Source: three-view drawing plus pictorial views. Frame: mm from the lowest corner of the part. A direction names the side the tool comes from. Give positions to 0.01 mm unless a question says otherwise; leave off trailing zeros. Loops run counter-clockwise (first coordinate to the right, second up) from the corner with the lowest first, then second, coordinate; pieces in that order, holes last. Notation, with made-up numbers: (-25.75, 75) - (-19.75, 75) arc R18 cw to (-19.75, 107) - close; hole circle Ø5 at (19, -17). An arc over 180 degrees is marked (long way). One line per item, written item: value.
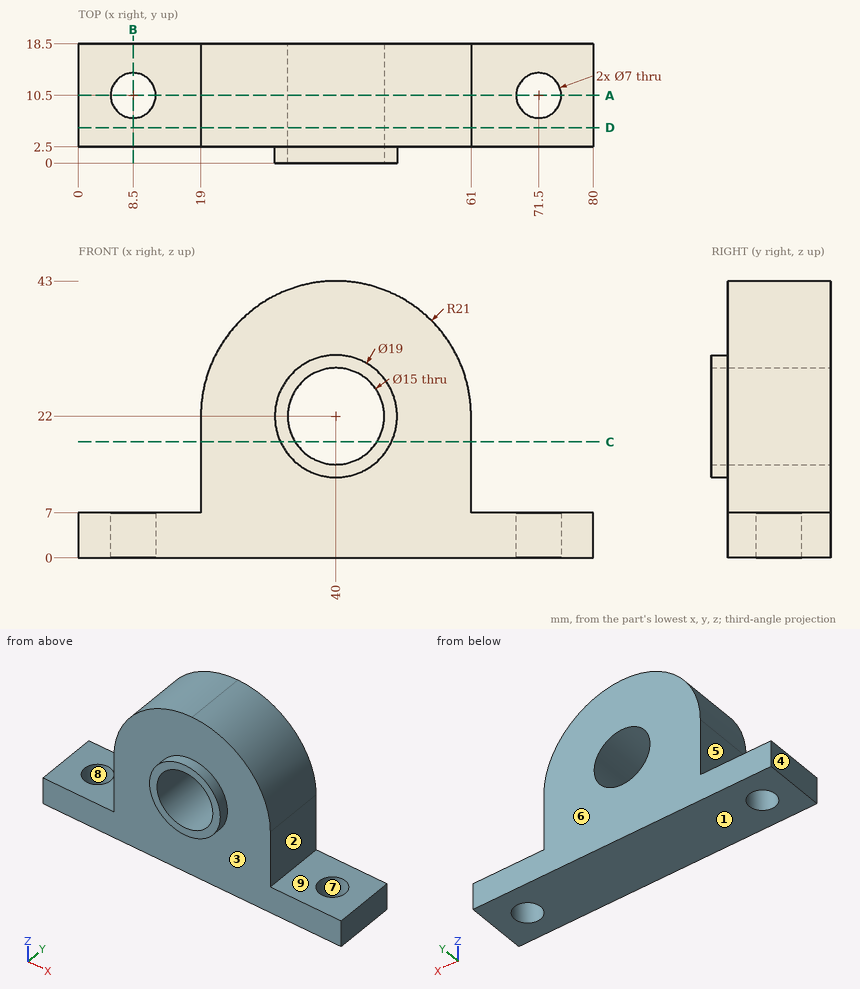
Item 1: Draft query along Y for the marked faces 6, 7, 8 and 9. Return one class per face: pulls with the +Y half, pulls with the -Y half, needs draft (parallel to the pull), parting line crosses it, or undercut.
Verdict:
face 6: pulls with the +Y half
face 7: undercut
face 8: undercut
face 9: needs draft
Item 2: Access query for the marked faces 1, 2, 3, 4 and 5. Directions: +Z, -Z, +X, -X, +Y, -Y. A direction counts if a zero-diameter tool reaches every point of the face in a straight line with its end or side. Return the directions, or none.
Verdict:
face 1: -Z, +X, -X, +Y, -Y
face 2: +Z, +X, +Y, -Y
face 3: -Y
face 4: +Z, -Z, -X, +Y, -Y
face 5: +Z, -X, +Y, -Y
Item 3: Pin query (flat end, axial travel): P1, Ø5.5, axis at x = 8.5, y = 10.5, coming from the -Z side; P2, Ø3, axis at x = 26, z = 38, coming from the -Y side; P3, Ø1, axis at x = 68, y = 11, coming from the +Z side; P4, Ø5, axis at y = 10, z = 19.5, coming from the +X side. Return the tip coordinate at first contact, or that it passes through.
Verdict:
P1: passes through
P2: stops at y = 2.5
P3: stops at z = 7
P4: stops at x = 61
Item 4: Section A-A, the plane y = 10.5. Output: boundary loops of the cut face in (x, z), and give its area (3 significant figures).
Verdict:
outline: (0, 0) - (5, 0) - (5, 7) - (0, 7) - close; (12, 0) - (68, 0) - (68, 7) - (61, 7) - (61, 22) arc R21 ccw to (40, 43) arc R21 ccw to (19, 22) - (19, 7) - (12, 7) - close; (75, 0) - (80, 0) - (80, 7) - (75, 7) - close; hole circle Ø15 at (40, 22)
area: 1,610 mm^2
Item 5: Section C-C, the plane z = 18. Output: boundary loops of the cut face in (x, y).
Verdict:
outline: (19, 2.5) - (31.38, 2.5) - (31.38, 0) - (33.66, 0) - (33.66, 18.5) - (19, 18.5) - close; (46.34, 0) - (48.62, 0) - (48.62, 2.5) - (61, 2.5) - (61, 18.5) - (46.34, 18.5) - close
Item 6: Material intervals for L1, parallel to Z at x = 40, y = 13.75; L2, parallel to X at y = 11.75, z = 3.5; L3, parallel to Y at x = 24, z = 23.5, sorted ascending.
Verdict:
L1: z = 0 to 14.5, 29.5 to 43
L2: x = 0 to 5.23, 11.77 to 68.23, 74.77 to 80
L3: y = 2.5 to 18.5
Item 7: Section D-D, the plane y = 5.5. Output: boundary loops of the cut face in (x, z).
Verdict:
outline: (0, 0) - (80, 0) - (80, 7) - (61, 7) - (61, 22) arc R21 ccw to (40, 43) arc R21 ccw to (19, 22) - (19, 7) - (0, 7) - close; hole circle Ø15 at (40, 22)
Item 8: Section B-B, the plane x = 8.5. Output: boundary loops of the cut face in (y, z), and give its area (3 significant figures).
Verdict:
outline: (2.5, 0) - (7, 0) - (7, 7) - (2.5, 7) - close; (14, 0) - (18.5, 0) - (18.5, 7) - (14, 7) - close
area: 63.0 mm^2
